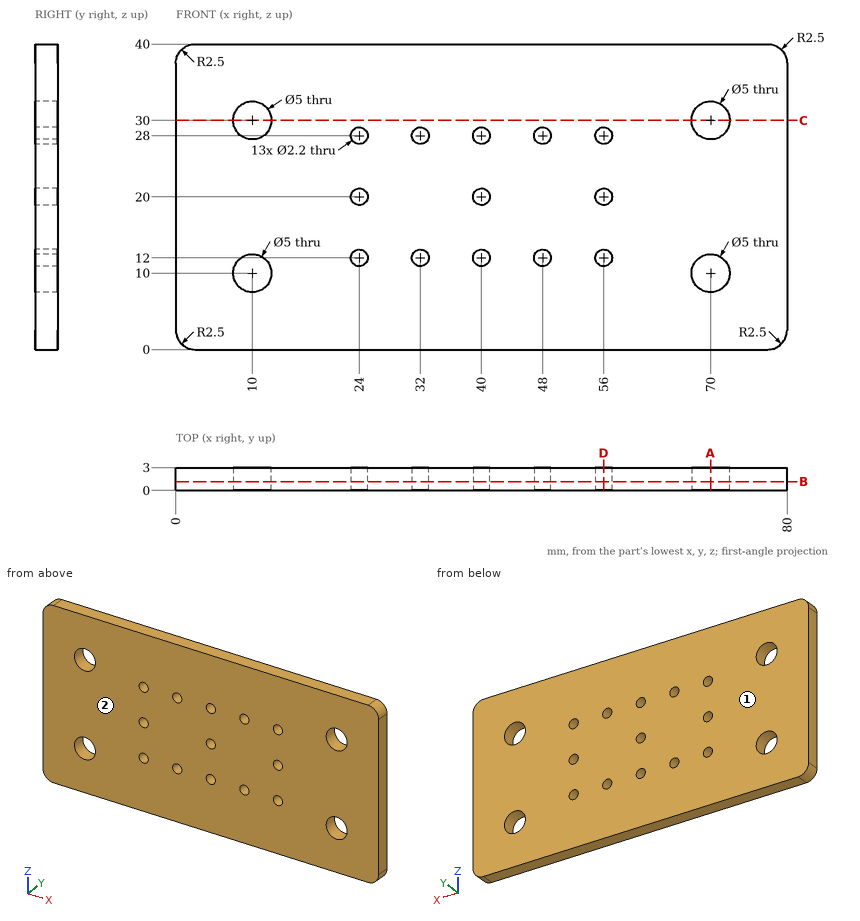
Geometry: see drawing. Coordinates: mm, zero at the bounding-box minimum. Round coordinates to 2 decimals unless told otherwise and drop trailing zeros. Write each loop counter-clockwise with the first axis right and the second up, starting at its lowest first coordinate (ties: lowest second). Pieces come first, ordered by that corner, then holes.
Item 1: Section query D-D (x = 56). Return loops of the section in (y, z).
Item 2: Mould query, pull axis Y, two halves, no side actions, for the marked faces 1 and 2. Classes: +Y half, -Y half, draft (parallel to the pull), parting line (faces both ways), or undercut.
Item 3: Section query B-B (y = 1.15). Give the number of separate pieces and of enclosed holes in the cut face, plus the area to 3 significant figures.
Item 4: Section query A-A (x = 70). Return loops of the section in (y, z).
Item 5: Section query C-C (z = 30). Return loops of the section in (x, y), plus the area to 3 significant figures.
Item 6: Material intervals for L1, parallel to Z at x = 24, y = 1.55; L2, parallel to X at y = 0.2, z = 30; L3, parallel to X at y = 1.6, z = 20, sorted ascending.
Item 7: Pin query (flat end, axial travel): P1, Ø5, axis at x = 43, z = 16.5, coming from the -Y side. Return the tip coordinate at first contact, or that it passes through.
Completed:
1. outline: (0, 0) - (3, 0) - (3, 10.9) - (0, 10.9) - close; (0, 13.1) - (3, 13.1) - (3, 18.9) - (0, 18.9) - close; (0, 21.1) - (3, 21.1) - (3, 26.9) - (0, 26.9) - close; (0, 29.1) - (3, 29.1) - (3, 40) - (0, 40) - close
2. face 1: +Y half
2. face 2: -Y half
3. separate pieces: 1
3. enclosed holes: 17
3. area: 3,070 mm2
4. outline: (0, 0) - (3, 0) - (3, 7.5) - (0, 7.5) - close; (0, 12.5) - (3, 12.5) - (3, 27.5) - (0, 27.5) - close; (0, 32.5) - (3, 32.5) - (3, 40) - (0, 40) - close
5. outline: (0, 0) - (7.5, 0) - (7.5, 3) - (0, 3) - close; (12.5, 0) - (67.5, 0) - (67.5, 3) - (12.5, 3) - close; (72.5, 0) - (80, 0) - (80, 3) - (72.5, 3) - close
5. area: 210 mm2
6. L1: z = 0 to 10.9, 13.1 to 18.9, 21.1 to 26.9, 29.1 to 40
6. L2: x = 0 to 7.5, 12.5 to 67.5, 72.5 to 80
6. L3: x = 0 to 22.9, 25.1 to 38.9, 41.1 to 54.9, 57.1 to 80
7. P1: stops at y = 0
